Work out the finished part from the listing and answer in its coordinate system (mm). A direction names the side the tool comes from. Coordinates: 2 decimals unless noted, no trailing zeros. Order: outer loops, then holes, each group sorted by start corner. A loop starts at its lowest first (then second) coordinate and runs counter-clockwise, first axis right, second up.
```python
from build123d import *

# Parameters (mm, degrees)
F1_DEPTH      = 25
F1_DEPTH_BACK = 25
F3_DEPTH      = 16.5
F3_DEPTH_BACK = 16.5
F4_DEPTH      = 8.4392210885
F4_DEPTH_BACK = 16.5
F6_D          = 5
F8_START      = -25
F8_DEPTH      = 50


with BuildPart() as f1:
    # F0 (on Right) → F1 (new body, two sides)
    with BuildSketch(Plane.YZ) as f1_sk:
        Polygon((3.0001489873, 6.5), (2.9994625902, 16.5), (0.4994625902, 16.5), (0.4994625902, 8.4392210885), (-6.5005374098, 8.4392210885), (-6.5005374098, 16.5), (-8.9995463506, 16.5), (-9.0002327559, 6.5), (-0.9999372788, -16.5), (9.0000627212, -16.5), align=None)
    extrude(amount=F1_DEPTH)
    extrude(f1_sk.sketch, amount=-F1_DEPTH_BACK)

    # F2 (on Top) → F3 (cut, two sides)
    with BuildSketch(Plane.XY) as f3_sk:
        Polygon((-3.5, 9.0000627212), (-6, 9.0000627212), (-6, 0.4994625902), (-3.5, 0.4994625902), (-3.5, 3.0001489873), align=None)
        Polygon((3.5, 9.0000627212), (-3.5, 9.0000627212), (-3.5, 3.0001489873), (-3.5, 0.4994625902), (3.5, 0.4994625902), (3.5, 3.0001489873), align=None)
        Polygon((6, 9.0000627212), (3.5, 9.0000627212), (3.5, 3.0001489873), (3.5, 0.4994625902), (6, 0.4994625902), align=None)
    extrude(amount=F3_DEPTH, mode=Mode.SUBTRACT)
    extrude(f3_sk.sketch, amount=-F3_DEPTH_BACK, mode=Mode.SUBTRACT)

    # F2 (on Top) → F4 (join, two sides)
    with BuildSketch(Plane.XY) as f4_sk:
        Polygon((-3.5, 9.0000627212), (-6, 9.0000627212), (-6, 0.4994625902), (-3.5, 0.4994625902), (-3.5, 3.0001489873), align=None)
        Polygon((6, 9.0000627212), (3.5, 9.0000627212), (3.5, 3.0001489873), (3.5, 0.4994625902), (6, 0.4994625902), align=None)
    extrude(amount=F4_DEPTH)
    extrude(f4_sk.sketch, amount=-F4_DEPTH_BACK)

    # F6 (through all)
    with Locations(Plane(origin=(0, 0, 0), x_dir=(1, 0, 0), z_dir=(0, 1, 0))):
        with Locations((0, -16.5018886328)):
            Hole(F6_D / 2)

    # F7 (on Front) → F8 (intersect)
    with BuildSketch(Plane.XZ.offset(F8_START)):
        Polygon((6.0645495541, -16.5), (25, 6.5), (25, 17.2385324479), (-25, 17.2385324479), (-25, 6.5), (-6.0119125992, -16.5), align=None)
    extrude(amount=F8_DEPTH, mode=Mode.INTERSECT)


solid = f1.part
```
1. The part is cut by section B-B (x = -10.5). Determine the outline of the cut face in (y, z), plus the area to 3 significant figures.
2. Flat-ended cylindrical pins translate along their axes: pin 1 (2 mm diameter, centred on x = 8.5, y = -2.5, fed in from +Z); pin 2 (4 mm diameter, centred on x = -2, z = 11.5, fed in from +Y); pin 3 (8 mm diameter, centred on x = 0.5, z = -6.5, fed in from -Y). Find the tip coordinate at first contact, or state that the pin passes through.
3. For faces 4 (the flat face through (16, 2, 16.5)), 5 (the flat face through (0, -6.501, 12)), 6 (the flat face through (3.5, 5, -4)), 7 (the flat face through (-15.64, 0.13, -4.84)), 8 (the flat face through (-13.256, 5.375, -2.605)), determine the directions among +Z, -Z, +X, -X, +Y, -Y from which every point of the face is accessible in a straight line to the end or side of a thin tool.
4. The part is cut by section A-A (z = 13). Determine the outline of the cut face in (x, y).
5. Consider probe 1 along X at (y, z) = (7.75, 7); probe 2 along Y at (x, z) = (-7, 14); probe 3 along X at (y, z) = (2, -2). Determine where each line is inside the solid, lowest interval first.
6. The part is cut by section C-C (z = -3). Determine the outline of the cut face in (x, y), plus the area to 3 significant figures.
7. The mould has two halves that part along X. Classify faces 1 (the flat face through (-14, -8, 16.5)), 2 (the flat face through (25, -3, 8)), 3 (the flat face through (-6, 2, 12)): released by +X, released by -X, zero draft, split by the parting line, or undercut.
8. The part is cut by section D-D (y = -5.75). Determine the outline of the cut face in (x, z).
Worked out:
1. outline: (-9, 6.5) - (-2.89, -11.06) - (7.58, -11.06) - (3, 6.5) - (3, 16.5) - (0.5, 16.5) - (0.5, 8.44) - (-6.5, 8.44) - (-6.5, 16.5) - (-9, 16.5) - close
1. area: 261 mm2
2. pin 1: stops at z = 8.44
2. pin 2: stops at y = -6.5
2. pin 3: stops at y = -5.87
3. face 4: +Z, +X, -X, +Y, -Y
3. face 5: +Z, +X, -X
3. face 6: +Z, -Z, +Y
3. face 7: -Z, -X, +Y, -Y
3. face 8: +Z, -X, +Y
4. outline: (-25, -9) - (25, -9) - (25, -6.5) - (-25, -6.5) - close; (-25, 0.5) - (-6, 0.5) - (-6, 3) - (-25, 3) - close; (6, 0.5) - (25, 0.5) - (25, 3) - (6, 3) - close
5. probe 1: x = -6 to -3.5, 3.5 to 6
5. probe 2: y = -9 to -6.5, 0.5 to 3
5. probe 3: x = -17.98 to -3.5, 3.5 to 18
6. outline: (-17.16, -5.7) - (17.18, -5.7) - (17.18, 5.48) - (6, 5.48) - (6, 9) - (3.5, 9) - (3.5, 0.5) - (-3.5, 0.5) - (-3.5, 9) - (-6, 9) - (-6, 5.48) - (-17.16, 5.48) - close
6. area: 366 mm2
7. face 1: zero draft
7. face 2: released by +X
7. face 3: undercut
8. outline: (-25, 6.5) - (-17.29, -2.84) - (17.31, -2.84) - (25, 6.5) - (25, 8.44) - (-25, 8.44) - close
